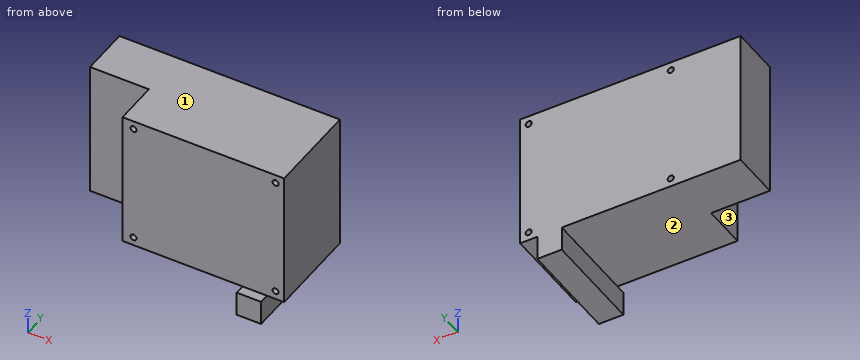
from build123d import *

# Parameters (mm, degrees)
SKETCH_1_W          = 90
SKETCH_1_H          = 56
EXTRUDE_1_DEPTH     = 20
SKETCH_4_W          = 66
SKETCH_4_H          = 56
EXTRUDE_3_DEPTH     = 18
SKETCH_2_R          = 1.25
CUT_EXTRUDE_1_DEPTH = 60
SKETCH_5_W          = 10
SKETCH_5_H          = 10
EXTRUDE_4_DEPTH     = 42


with BuildPart() as part:
    # 草图1 → 凸台-拉伸1 (new body)
    with BuildSketch(Plane(origin=(0, 0, 0), x_dir=(1, 0, 0), z_dir=(0, 1, 0))):
        Rectangle(SKETCH_1_W, SKETCH_1_H)
    extrude(amount=EXTRUDE_1_DEPTH)

    # 草图4 → 凸台-拉伸3 (add)
    with BuildSketch(Plane.XZ):
        with Locations((12, 0)):
            Rectangle(SKETCH_4_W, SKETCH_4_H)
    extrude(amount=EXTRUDE_3_DEPTH)

    # 草图2 → 切除-拉伸1 (cut)
    with BuildSketch(Plane(origin=(0, 20, 0), x_dir=(1, 0, 0), z_dir=(0, 1, 0))):
        with Locations(Location((41.5, 24.5, 0), (0, 0, 270))):
            Circle(SKETCH_2_R)
        with Locations(Location((41.5, -24.5, 0), (0, 0, 90))):
            Circle(SKETCH_2_R)
        with Locations(Location((-16.5, -24.5, 0), (0, 0, 270))):
            Circle(SKETCH_2_R)
        with Locations(Location((-16.5, 24.5, 0), (0, 0, 90))):
            Circle(SKETCH_2_R)
    extrude(amount=-CUT_EXTRUDE_1_DEPTH, mode=Mode.SUBTRACT)

    # 草图5 → 凸台-拉伸4 (add)
    with BuildSketch(Plane(origin=(0, 20, 0), x_dir=(1, 0, 0), z_dir=(0, 1, 0))):
        with Locations((33, 33)):
            Rectangle(SKETCH_5_W, SKETCH_5_H)
    extrude(amount=-EXTRUDE_4_DEPTH)


solid = part.part
Can you work these out from the model? Positions are in its coordinate system, mm. Face numbers are marked on the shaded views. A direction names the side the tool comes from. Coordinates: 2 decimals unless noted, no trailing zeros. Write each loop counter-clockwise with the first axis right and the second up, starting at its lowest first coordinate (ties: lowest second). Pieces come first, ordered by that corner, then holes. Notation, with made-up numbers: (-20.75, 21) - (-2.75, 21) arc R17 ccw to (-2.75, 51) - close; hole circle Ø11 at (3, 1). An arc over 180 degrees is marked (long way). Return JSON: item names as keys, results as strings. Group by question number.
Item 1: I'm going to push flat-ended pins straight in: pin 1 Ø19 at (x, y) = (-2, -8.5) entering from -Z; pin 2 Ø2 at (x, y) = (34.5, -20) entering from +Z; pin 3 Ø4 at (x, z) = (-16.5, 24.5) entering from -Y; pin 4 Ø1.5 at (x, z) = (41.5, -24.5) entering from +Y. Where does each tip first touch, or does it pass through?
Item 2: If we section it at B-B (z = 24.5): Write out the boundary of the cut face in (x, y).
Item 3: If we section it at C-C (y = 14): Write out the boundary of the cut face in (x, z).
Item 4: If we section it at A-A (x = -16.5): Write out the boundary of the cut face in (y, z), then the cut area to 3 significant figures.
Item 5: Please list where these lines run through material, in increasing order: probe 1 along X at (y, z) = (-6.5, -24.5); probe 2 along X at (y, z) = (1.5, -24.5); probe 3 along Z at (x, y) = (-15.5, -14).
Item 6: If we section it at D-D (z = -20): Write out the boundary of the cut face in (x, y).
Item 7: Which directions (+Z, -Z, +X, -X, +Y, -Y) give clear straight access to the entire face, cutting with the end or side of a thin tool? Please do the marked faces 1, 2 and 3.
Return value:
{
 "1": {"pin 1": "stops at z = -28", "pin 2": "stops at z = -28", "pin 3": "stops at y = -18", "pin 4": "passes through"},
 "2": {"outline": "(-45, 0) - (-21, 0) - (-21, -18) - (-17.75, -18) - (-17.75, 20) - (-45, 20) - close; (-15.25, -18) - (40.25, -18) - (40.25, 20) - (-15.25, 20) - close; (42.75, -18) - (45, -18) - (45, 20) - (42.75, 20) - close"},
 "3": {"outline": "(-45, -28) - (28, -28) - (28, -38) - (38, -38) - (38, -28) - (45, -28) - (45, 28) - (-45, 28) - close; hole circle Ø2.5 at (-16.5, -24.5); hole circle Ø2.5 at (-16.5, 24.5); hole circle Ø2.5 at (41.5, -24.5); hole circle Ø2.5 at (41.5, 24.5)"},
 "4": {"outline": "(-18, -28) - (20, -28) - (20, -25.75) - (-18, -25.75) - close; (-18, -23.25) - (20, -23.25) - (20, 23.25) - (-18, 23.25) - close; (-18, 25.75) - (20, 25.75) - (20, 28) - (-18, 28) - close", "area": "1,940 mm^2"},
 "5": {"probe 1": "x = -21 to -17.75, -15.25 to 40.25, 42.75 to 45", "probe 2": "x = -45 to -17.75, -15.25 to 40.25, 42.75 to 45", "probe 3": "z = -28 to -25.25, -23.75 to 23.75, 25.25 to 28"},
 "6": {"outline": "(-45, 0) - (-21, 0) - (-21, -18) - (45, -18) - (45, 20) - (-45, 20) - close"},
 "7": {"face 1": "+Z, +X, -X, +Y, -Y", "face 2": "-Z, -X, +Y, -Y", "face 3": "+Z, -Z, -X, -Y"}
}
